Can you work these out from the drawing? Everything is in mm from the part's minimum corner. A direction names the side the tool comes from. Give positions to 0.01 mm unless a question says otherwise; leave off trailing zeros. Loops run counter-clockwise (first coordinate to the right, second up) from the corner with the lowest first, then second, coordinate; pieces in that order, holes last. Notation, with made-up numbers: (41.5, -39) -> (50.5, -39) arc R18 ccw to (50.5, -30) -> close; hole circle Ø1 at (45.5, -18.75). An arc over 180 degrees is marked (long way). Write item = value, one per line. Start each with the question number.
1) I'm going to push flat-ended pins straight in: pin 1 Ø8 at (x, y) = (22, 32) entering from +Z; pin 2 Ø8 at (x, y) = (11.5, 49) entering from +Z; pin 3 Ø2 at (y, z) = (42, 20.5) entering from -X; pin 4 Ø10 at (x, z) = (28, 17) entering from +Y. Where does each tip first touch, or does it pass through?
2) I want a section at D-D (y = 9). List the corners of the cut face in (x, z) for me.
3) On a 3-axis mill with a long thin cutter (end or side, diameter ignored), from which of +Z, -Z, +X, -X, +Y, -Y can I reach the whole of each face in a straight line? I mean the marked faces 1 and 2. Say none if no direction works.
4) I want a section at A-A (x = 19.5). List the corners of the cut face in (y, z) for me.
5) I want a section at B-B (z = 19.5). List the corners of the cut face in (x, y) for me, and give its area (3 significant figures).
6) If we mould it in two halves opening along Z, with no side actions, what happens to the marked faces 3 and 4? For each: +Z half, -Z half, draft (parallel to the pull), parting line (faces both ways), or undercut.
7) I want a section at C-C (y = 39). List the corners of the cut face in (x, z) for me, and give its area (3 significant figures).
8) I need wall thicknesses on probe 1 along Y at (x, z) = (33, 26.5); probe 2 along Y at (x, z) = (28.5, 34.5); probe 3 along Z at (x, y) = (20, 54). Which ranges of each line are inside material? Lowest first, please. Write a range as from..to.
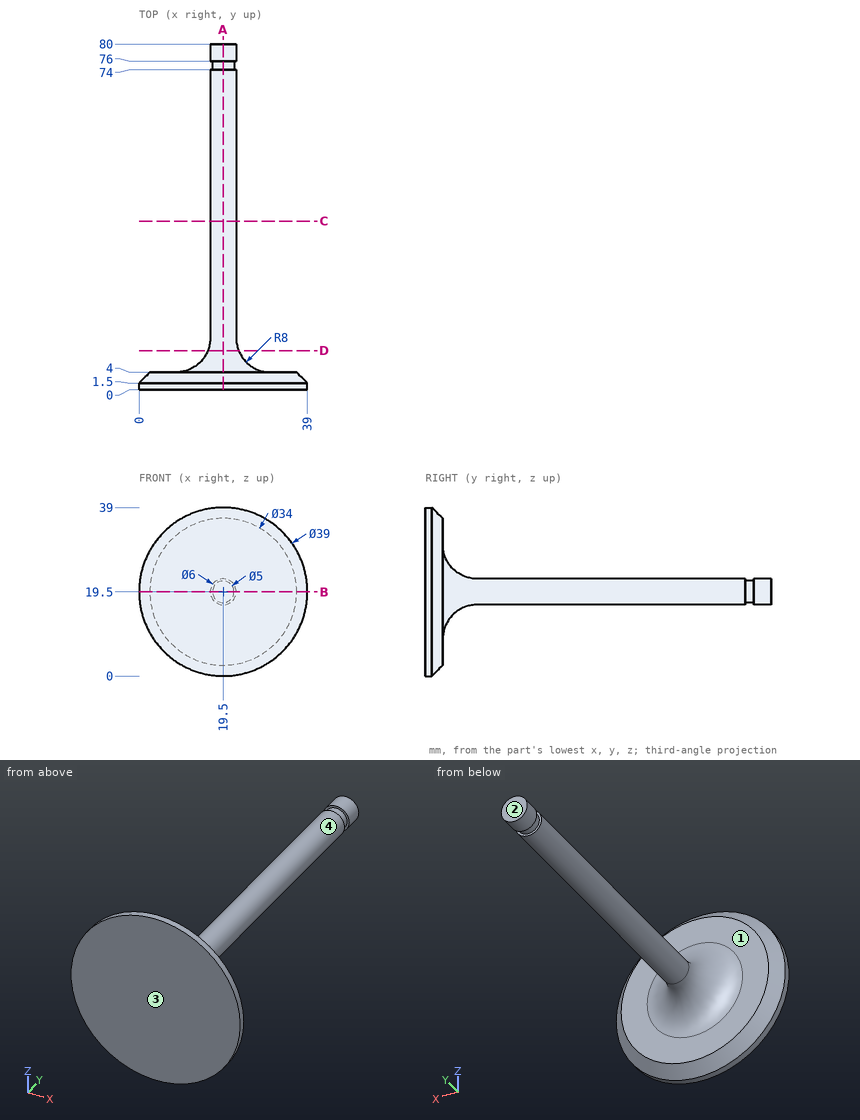
Answer list:
q1.pin_1 = 22.5
q1.pin_2 = through
q1.pin_3 = 16.5
q1.pin_4 = 8.39
q2.outline = circle Ø7.17 at (19.5, 19.5)
q3.face_1 = +Y
q3.face_2 = +Z, -Z, +X, -X, +Y
q4.outline = (0, 0) -> (1.5, 0) -> (4, 2.5) -> (4, 8.5) arc R8 cw to (12, 16.5) -> (74, 16.5) -> (74, 17) -> (76, 17) -> (76, 16.5) -> (80, 16.5) -> (80, 22.5) -> (76, 22.5) -> (76, 22) -> (74, 22) -> (74, 22.5) -> (12, 22.5) arc R8 cw to (4, 30.5) -> (4, 36.5) -> (1.5, 39) -> (0, 39) -> close
q5.outline = (0, 0) -> (39, 0) -> (39, 1.5) -> (36.5, 4) -> (30.5, 4) arc R8 cw to (22.5, 12) -> (22.5, 74) -> (22, 74) -> (22, 76) -> (22.5, 76) -> (22.5, 80) -> (16.5, 80) -> (16.5, 76) -> (17, 76) -> (17, 74) -> (16.5, 74) -> (16.5, 12) arc R8 cw to (8.5, 4) -> (2.5, 4) -> (0, 1.5) -> close
q5.area = 631 mm^2
q6.face_3 = draft
q6.face_4 = parting line
q7.outline = circle Ø6 at (19.5, 19.5)
q7.area = 28.3 mm^2
q8.probe_1 = 0..4
q8.probe_2 = 0..3.51
q8.probe_3 = 16.54..22.46
